Work out the finished part from the listing and answer in its coordinate system (mm). A direction names the side the tool comes from. Round coordinates to 2 decimals unless told otherwise and drop trailing zeros. Order: outer loops, then holes, each group sorted by start corner. A loop starts at its lowest first (then second) coordinate and runs counter-clockwise, first axis right, second up. Notation, with made-up numbers: (-16.5, 45) -> (-6.5, 45) arc R28 ccw to (-6.5, 67) -> close; hole circle Ø3 at (-15.5, 85). An arc over 180 degrees is marked (long way). Use a Markdown table: item, result. Add a question column.
Item 1: A cutting plane is placed at B-B, the plane x = 4.5. Determine the outline of the cut face in (y, z), plus the area to 3 significant figures.
Item 2: Flat-ended cylindrical pins translate along their axes: P1, Ø1.5, axis at y = 4.5, z = 0, coming from the +X side; P2, Ø3, axis at x = 21.5, y = 2.5, coming from the -Z side; P3, Ø1.5, axis at x = 6.5, z = -3.5, coming from the +Y side. Find the tip coordinate at first contact, or state that the pin passes through.
Item 3: Find the intervals of material crossed by L1, parallel to Z at x = -0.1, y = 0; L2, parallel to Z at x = 0.7, y = 0; L3, parallel to Y at x = 0.5, z = 1.5, in increasing order. Write a range as [from, to].
Item 4: For a pull along Z with two mould halves and no side action, classify faces 4 (the cylindrical face through (-2.129, -5.158, 3.955)), 5 (the flat face through (-3.4, -1.5, -2.6)), 6 (the flat face through (-5, -2.5, 2.5)), 7 (the cylindrical face through (0, 0, -2)) as +Z half, -Z half, draft (parallel to the pull), parting line (faces both ways), or undercut.
Item 5: A cutting plane is placed at A-A, the plane x = -3. Determine the outline of the cut face in (y, z), plus the area to 3 significant figures.
Item 6: A tool of negligible diameter and unlimited length cuts with its end or side. For faces 1 (the flat face through (-3.4, -1.5, 2.6)), 2 (the flat face through (0, 3, 3)), 3 (the flat face through (30, 0, 0)), from which of +Z, -Z, +X, -X, +Y, -Y can it reach the whole face along a straight path? Write none if from no direction.
Autodesk Inventor part; units mm, degrees
ref_plane "Work Plane1" through (15, 0, 0) normal (0, 0.5, 0.866) x (1, 0, 0)
ref_plane "YZ Plane" through (0, 0, 0) normal (1, 0, 0) x (0, 1, 0)
ref_plane "XZ Plane" through (0, 0, 0) normal (0, 1, 0) x (-1, 0, 0)
sketch "Schizzo1" plane through (0, 0, 0) normal (0, 0, 1) x (1, 0, 0)
  line L0 (2.6547, 0) -> (30, 0)
  line L1 (30, 0) -> (30, 4)
  line L2 (30, 4) -> (0, 4)
  line L3 (0, 4) -> (0, 6.5)
  line L4 (0, 6.5) -> (-5, 6.5)
  line L5 (-5, 6.5) -> (-5, 3.4641)
  line L6 (-5, 3.4641) -> (-2, 3.4641)
  line L7 (-2, 3.4641) -> (-1.1547, 2)
  line L8 (-12, 0) -> (37, 0)
  line L9 (0, -1.3) -> (0, 7.8)
  line L10 (-1.1547, 2) -> (1.5, 2)
  line L11 (1.5, 2) -> (2.6547, 0)
  line L12 (-5, 3.4641) -> (-5, 0) construction
  line L13 (-5, 5.7) -> (-4.2, 6.5)
  dimension "d0" = 5
  dimension "d1" = 3
  dimension "d2" = 60
  dimension "d3" = 8
  dimension "d4" = 6.9282
  dimension "d5" = 13
  dimension "d15" = 6.5
  dimension "d16" = 4
  dimension "d17" = 30
  dimension "d32" = 45
  dimension "d33" = 0.8
revolve "Corpo" add sketch "Schizzo1" angle 360 about axis through (2.6547, 0, 0) along (1, 0, 0) contours L11 L10 L9 L2 L1 L0 | L10 L7 L6 L5 L13 L4 L3 L9 | L13 L5 L4
revolve "Smusso2" cut sketch "Schizzo1" angle 360 about axis through (-10, 0, 0) along (1, 0, 0) contours L13 L5 L4
sketch "Schizzo2" plane through (-5, 0, 0) normal (-1, 0, 0) x (0, 0, 1)
  circle A0 centre (0, 0) radius 3.4641
  line L0 (0, -9.1) -> (0, 9.1)
  line L1 (-9.1, 0) -> (9.1, 0)
  line L2 (3.4641, 0) -> (1.7321, -3)
  line L3 (1.7321, -3) -> (-1.7321, -3)
  line L4 (-1.7321, -3) -> (-3.4641, 0)
  line L5 (-3.4641, 0) -> (-1.7321, 3)
  line L6 (-1.7321, 3) -> (1.7321, 3)
  line L7 (1.7321, 3) -> (3.4641, 0)
  point P0 (0, 0)
extrude "Intaglio" add sketch "Schizzo2" against normal up to next contours L7 A0 | A0 L2 | L6 L0 A0 | A0 L0 L3 | L0 L6 A0 | A0 L3 L0 | L4 A0 | A0 L5
thread "Filettatura"
chamfer "Smusso1" distance 0.7668 distance2 0.7668 1 edges at (30, -4, 0) measured on face at (30, -0.4013, -0.6579)
ref_plane "Work Plane1" through (15, 0, 0) normal (0, 0.5, 0.866) x (1, 0, 0)
equation "\"d0\" = KOH"
equation "\"d1\" = INTI"
equation "\"d3\" = GD"
equation "\"d4\" = 1.1547 * SW"
equation "\"d5\" = KOD"
equation "\"d15\" = INFT"
equation "\"d16\" = SDT"
equation "\"d17\" = NLG"
equation "\"d33\" = Cham"
equation "\"d7\" = GEL"
equation "\"d9\" = -0.5 * SPD + 0.5 * GD"
equation "\"d12\" = GUL"
equation "\"GD\" = NND"
equation "\"NLG\" = 30"
equation "\"GEL\" = 23"
equation "\"KOD\" = 13"
equation "\"KOH\" = 5"
equation "\"GUL\" = 0.61345 * PTC"
equation "\"SW\" = 6"
equation "\"INTI\" = 3"
equation "\"SPD\" = NND - 1.2269 * PTC"
equation "\"SDT\" = 4"
equation "\"INFT\" = 6.5"
equation "\"Cham\" = 0.8"
equation "\"TOA\" = 30deg"
equation "\"GD1\" = THREADDIA - 1.2269 * PTC"
equation "\"THREADDIA\" = 8"
equation "\"BDM\" = NND"
equation "\"FAWI\" = 45deg"
equation "\"RR\" = 0.1 * NND"
equation "\"PTC\" = 1.25"
equation "\"NND\" = 8"
equation "\"FAWI1\" = 45deg"
equation "\"GAL\" = 0.61345 * PTC"
equation "\"E0\" = 1.155 * SW"
properties part number "DIN 6912 - M8 x 30" material "Acciaio, Dolce"
Reported:
| question | item | result |
|---|---|---|
| 1 | outline | circle Ø8 at (0, 0) |
| 1 | area | 50.3 mm² |
| 2 | P1 | x = 29.48 |
| 2 | P2 | z = -3.87 |
| 2 | P3 | y = 2.9 |
| 3 | L1 | [-6.5, -2], [2, 6.5] |
| 3 | L2 | [-4, -2], [2, 4] |
| 3 | L3 | [-3.71, -1.32], [1.32, 3.71] |
| 4 | face 4 | parting line |
| 4 | face 5 | undercut |
| 4 | face 6 | draft |
| 4 | face 7 | undercut |
| 5 | outline | circle Ø13 at (0, 0); hole (-3, -1.73) -> (0, -3.46) -> (3, -1.73) -> (3, 1.73) -> (0, 3.46) -> (-3, 1.73) -> close |
| 5 | area | 102 mm² |
| 6 | face 1 | -X |
| 6 | face 2 | +X |
| 6 | face 3 | +Z, -Z, +X, +Y, -Y |
